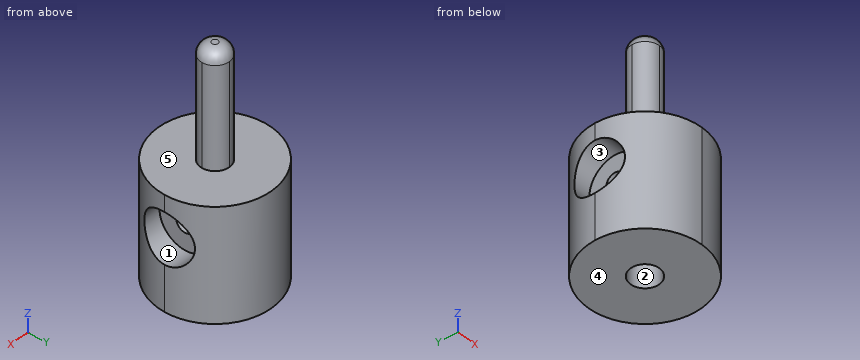
from build123d import *

# Parameters (mm, degrees)
F1_DEPTH  = 10
F2_DEPTH  = 10
F4_R      = 1.2735627731
F5_DEPTH  = 8
F6_R      = 0.75
F7_DEPTH  = 12.5
F9_R      = 2.25
F9_R_2    = 0.75
F10_DEPTH = 2
F12_R     = 2.25
F12_R_2   = 0.75
F13_DEPTH = 2


# Not quite as in the source:
# - a fillet or chamfer that OpenCascade refuses, or shapes differently, is made with other operations: its cross-section is extruded or revolved along the edge and cut away or added
# - a feature names something its author has since deleted; it is built from what else it names


with BuildPart() as f1:
    # F0 (on Top) → F1 (new body)
    with BuildSketch(Plane.XY):
        with BuildLine():
            Line((0, 0), (1.2735627731, 0))
            ThreePointArc((1.2735627731, 0), (0.9005448731, 0.9005448731), (0, 1.2735627731))
            Line((0, 1.2735627731), (0, 0))
        make_face()
        with BuildLine():
            Line((0, 0), (0, 1.2735627731))
            ThreePointArc((0, 1.2735627731), (-0.9005448731, 0.9005448731), (-1.2735627731, 0))
            Line((-1.2735627731, 0), (0, 0))
        make_face()
        with BuildLine():
            ThreePointArc((-1.2735627731, 0), (-0.9005448731, -0.9005448731), (0, -1.2735627731))
            Line((0, -1.2735627731), (0, 0))
            Line((0, 0), (-1.2735627731, 0))
        make_face()
        with BuildLine():
            ThreePointArc((0, -1.2735627731), (0.9005448731, -0.9005448731), (1.2735627731, 0))
            Line((1.2735627731, 0), (0, 0))
            Line((0, 0), (0, -1.2735627731))
        make_face()
    extrude(amount=F1_DEPTH)

    # F0 (on Top) → F2 (join)
    with BuildSketch(Plane.XY):
        with BuildLine():
            ThreePointArc((0.0602184818, -5.0337774218), (3.5808999931, -3.5383183346), (5.0341376022, 0))
            ThreePointArc((5.0341376022, 0), (-0.0301919188, 5.0340470643), (-5.033775454, -0.0603827516))
            ThreePointArc((-5.033775454, -0.0603827516), (-3.5167784797, -3.6020564297), (0.0602184818, -5.0337774218))
        make_face()
        with BuildLine():
            ThreePointArc((0, 1.2735627731), (0.9005448731, 0.9005448731), (1.2735627731, 0))
            ThreePointArc((1.2735627731, 0), (0.9005448731, -0.9005448731), (0, -1.2735627731))
            ThreePointArc((0, -1.2735627731), (-0.9005448731, -0.9005448731), (-1.2735627731, 0))
            ThreePointArc((-1.2735627731, 0), (-0.9005448731, 0.9005448731), (0, 1.2735627731))
        make_face(mode=Mode.SUBTRACT)
        with BuildLine():
            Line((0, 0), (1.2735627731, 0))
            ThreePointArc((1.2735627731, 0), (0.9005448731, 0.9005448731), (0, 1.2735627731))
            Line((0, 1.2735627731), (0, 0))
        make_face()
        with BuildLine():
            Line((0, 0), (0, 1.2735627731))
            ThreePointArc((0, 1.2735627731), (-0.9005448731, 0.9005448731), (-1.2735627731, 0))
            Line((-1.2735627731, 0), (0, 0))
        make_face()
        with BuildLine():
            ThreePointArc((-1.2735627731, 0), (-0.9005448731, -0.9005448731), (0, -1.2735627731))
            Line((0, -1.2735627731), (0, 0))
            Line((0, 0), (-1.2735627731, 0))
        make_face()
        with BuildLine():
            ThreePointArc((0, -1.2735627731), (0.9005448731, -0.9005448731), (1.2735627731, 0))
            Line((1.2735627731, 0), (0, 0))
            Line((0, 0), (0, -1.2735627731))
        make_face()
    extrude(amount=-F2_DEPTH)

    # F3: fillet of radius 1 on 1 edges, made by hand

    # F3_s1 → F3_t2 (revolve, cut)
    with BuildSketch(Plane.YZ):
        with BuildLine():
            ThreePointArc((-1.2735627731, 9), (-0.9806695543, 9.7071067812), (-0.2735627731, 10))
            Line((-0.2735627731, 10), (-1.2735627731, 10))
            Line((-1.2735627731, 10), (-1.2735627731, 9))
        make_face()
    revolve(axis=Axis((0, 0, 10), (0, 0, 1)), mode=Mode.SUBTRACT)

    # F4 (on face) → F5 (cut)
    with BuildSketch(Plane(origin=(0, 0, -10), x_dir=(1, 0, 0), z_dir=(0, 0, -1))):
        Circle(F4_R)
    extrude(amount=-F5_DEPTH, mode=Mode.SUBTRACT)

    # F6 (on Right) → F7 (cut, symmetric)
    with BuildSketch(Plane.YZ):
        with Locations((0, -3.7172080483)):
            Circle(F6_R)
    extrude(amount=F7_DEPTH, both=True, mode=Mode.SUBTRACT)

    # F9 (on offset) → F10 (cut, symmetric)
    with BuildSketch(Plane.YZ.offset(5)):
        with Locations((0, -3.7172080483)):
            Circle(F9_R)
        with Locations((0, -3.7172080483)):
            Circle(F9_R_2, mode=Mode.SUBTRACT)
    extrude(amount=F10_DEPTH, both=True, mode=Mode.SUBTRACT)

    # F12 (on offset) → F13 (cut, symmetric)
    with BuildSketch(Plane.YZ.offset(-5)):
        with Locations((0, -3.7172080483)):
            Circle(F12_R)
        with Locations((0, -3.7172080483)):
            Circle(F12_R_2, mode=Mode.SUBTRACT)
    extrude(amount=F13_DEPTH, both=True, mode=Mode.SUBTRACT)


solid = f1.part
Work out the finished part from the listing and answer in its coordinate system (mm). Face numbers are marked on the shaded views. A direction names the side the tool comes from. Coordinates: 2 decimals unless noted, no trailing zeros. Loops run counter-clockwise (first coordinate to the right, second up) from the corner with the lowest first, then second, coordinate; pieces in that order, holes last. Notation, with made-up numbers: M 42,31.25 L 69,31.25 A15 ccw 69,58.25 Z; hole C 14.25,-13 d4. An arc over 180 degrees is marked long. Answer in a Markdown table with one row per item. Add a question column.
1. Flat-ended cylindrical pins translate along their axes: P1, Ø2, axis at y = -0.5, z = -3.5, coming from the -X side; P2, Ø5, axis at x = -3, z = 7.5, coming from the +Y side; P3, Ø4, axis at y = 0, z = -3.72, coming from the +X side. Find the tip coordinate at first contact, or state that the pin passes through.
2. Find section B-B, the plane y = 0.5. State how many separate pieces and enclosed holes the cut face has, then the cut area to 3 significant figures.
3. Find section D-D, the plane y = -1.5. Write down the section's boundary in (x, z).
4. The mould has two halves that part along Z. Classify the marked faces 3, 4 and 5: pulls with the +Z half, pulls with the -Z half, needs draft (parallel to the pull), parting line crosses it, or undercut.
5. Find section C-C, the plane z = 2.25. Write down the section's boundary in (x, y), then the cut area to 3 significant figures.
6. A tool of negligible diameter and unlimited length cuts with its end or side. For the marked faces 1 and 2, from which of +Z, -Z, +X, -X, +Y, -Y can it reach the whole face along a straight path? Write none if from no direction.
7. Consider L1, parallel to Z at x = -3.45, y = 0; L2, parallel to Z at x = -2, y = 0; L3, parallel to Z at x = -1.5, y = 4. Determine where each line is inside the solid, lowest interval first.
8. Find section A-A, the plane x = -2.5. Write down the section's boundary in (y, z), then the cut area to 3 significant figures.
Reported:
| question | item | result |
|---|---|---|
| 1 | P1 | stops at x = -3 |
| 1 | P2 | stops at y = 1.17 |
| 1 | P3 | stops at x = 3 |
| 2 | separate pieces | 3 |
| 2 | enclosed holes | 0 |
| 2 | area | 82.6 mm^2 |
| 3 | outline | M -4.81,-10 L 4.81,-10 L 4.81,-5.39 L 3,-5.39 L 3,-2.04 L 4.81,-2.04 L 4.81,0 L -4.81,0 L -4.81,-2.04 L -3,-2.04 L -3,-5.39 L -4.81,-5.39 Z |
| 4 | face 3 | undercut |
| 4 | face 4 | pulls with the -Z half |
| 4 | face 5 | pulls with the +Z half |
| 5 | outline | C 0,0 d2.55 |
| 5 | area | 5.10 mm^2 |
| 6 | face 1 | +X |
| 6 | face 2 | -Z |
| 7 | L1 | z = -10 to -5.97, -1.47 to 0 |
| 7 | L2 | z = -10 to -4.47, -2.97 to 0 |
| 7 | L3 | z = -10 to 0 |
| 8 | outline | M -4.37,-10 L 4.37,-10 L 4.37,0 L -4.37,0 Z; hole C 0,-3.72 d1.5 |
| 8 | area | 85.6 mm^2 |
